```python
from build123d import *

# Parameters (mm, degrees)
AUFSATZ_LINEAR_AUSTRAGEN1_DEPTH      = 3
AUFSATZ_LINEAR_AUSTRAGEN1_DEPTH_BACK = 1
AUFSATZ_LINEAR_AUSTRAGEN3_DEPTH      = 31.65
SCHNITT_LINEAR_AUSTRAGEN1_DEPTH      = 28.65
SKIZZE7_R                            = 2.5
SCHNITT_LINEAR_AUSTRAGEN2_DEPTH      = 110.867294952
SCHNITT_LINEAR_AUSTRAGEN6_DEPTH      = 2
SKIZZE9_R                            = 1
SCHNITT_LINEAR_AUSTRAGEN5_DEPTH      = 13.1
SKIZZE10_R                           = 1.25
SCHNITT_LINEAR_AUSTRAGEN7_DEPTH      = 111.405717696
SKIZZE11_R                           = 2.75
SCHNITT_LINEAR_AUSTRAGEN8_DEPTH      = 1.4


with BuildPart() as part:
    # Skizze2 → Aufsatz-Linear austragen1 (new, two sides: drawn at the far end of the back side and taken through both)
    with BuildSketch(Plane(origin=(0, 0, 0), x_dir=(1, 0, 0), z_dir=(0, 1, 0)).offset(-AUFSATZ_LINEAR_AUSTRAGEN1_DEPTH_BACK)):
        Polygon((-53.033008589, 53.033008589), (0, 0), (53.033008589, 53.033008589), (0, 75), align=None)
        Polygon((53.033008589, 53.033008589), (0, 0), (75, 0), align=None)
        Polygon((75, 0), (0, 0), (53.033008589, -53.033008589), align=None)
        Polygon((53.033008589, -53.033008589), (0, 0), (-53.033008589, -53.033008589), (0, -75), align=None)
        Polygon((-53.033008589, 53.033008589), (-75, 0), (0, 0), align=None)
        Polygon((0, 0), (-75, 0), (-53.033008589, -53.033008589), align=None)
    extrude(amount=AUFSATZ_LINEAR_AUSTRAGEN1_DEPTH + AUFSATZ_LINEAR_AUSTRAGEN1_DEPTH_BACK)

    # Skizze5 → Aufsatz-Linear austragen3 (add)
    with BuildSketch(Plane(origin=(0, 0, 0), x_dir=(1, 0, 0), z_dir=(0, 1, 0))):
        Polygon((20.35, -4), (28.35, -4), (28.35, -11.925), (-28.35, -11.925), (-28.35, 11.925), (28.35, 11.925), (28.35, 4), (20.35, 4), (20.35, 9.925), (-20.35, 9.925), (-20.35, -9.925), (20.35, -9.925), align=None)
    extrude(amount=AUFSATZ_LINEAR_AUSTRAGEN3_DEPTH)

    # Skizze6 → Schnitt-Linear austragen1 (cut)
    with BuildSketch(Plane.XY.offset(11.925)):
        Polygon((-19, 31.65), (19, 31.65), (-2.152730863, 14.994542406), align=None)
    extrude(amount=-SCHNITT_LINEAR_AUSTRAGEN1_DEPTH, mode=Mode.SUBTRACT)

    # Skizze7 → Schnitt-Linear austragen2 (cut, through all)
    with BuildSketch(Plane(origin=(0, 3, 0), x_dir=(1, 0, 0), z_dir=(0, 1, 0))):
        with Locations(Location((35, 40, 0), (0, 0, 270))):
            Circle(SKIZZE7_R)
        with Locations(Location((-35, 40, 0), (0, 0, 270))):
            Circle(SKIZZE7_R)
        with Locations(Location((0, -40, 0), (0, 0, 270))):
            Circle(SKIZZE7_R)
    extrude(amount=-SCHNITT_LINEAR_AUSTRAGEN2_DEPTH, mode=Mode.SUBTRACT)

    # Skizze8 → Schnitt-Linear austragen6 (cut)
    with BuildSketch(Plane(origin=(0, 3, 0), x_dir=(1, 0, 0), z_dir=(0, 1, 0))):
        Polygon((-32.35, 8.05), (-32.35, -8.05), (-49.95, 0), align=None)
        Polygon((32.35, -8.05), (49.95, 0), (32.35, 8.05), align=None)
    extrude(amount=-SCHNITT_LINEAR_AUSTRAGEN6_DEPTH, mode=Mode.SUBTRACT)

    # Skizze9 → Schnitt-Linear austragen5 (cut)
    with BuildSketch(Plane(origin=(0, 31.65, 0), x_dir=(1, 0, 0), z_dir=(0, 1, 0))):
        with Locations(Location((-24.4, -5.375, 0), (0, 0, 270))):
            Circle(SKIZZE9_R)
        with Locations(Location((-24.4, 5.525, 0), (0, 0, 270))):
            Circle(SKIZZE9_R)
        with Locations(Location((24.9, 5.525, 0), (0, 0, 270))):
            Circle(SKIZZE9_R)
        with Locations(Location((24.9, -5.375, 0), (0, 0, 270))):
            Circle(SKIZZE9_R)
    extrude(amount=-SCHNITT_LINEAR_AUSTRAGEN5_DEPTH, mode=Mode.SUBTRACT)

    # Skizze10 → Schnitt-Linear austragen7 (cut, through all)
    with BuildSketch(Plane(origin=(0, 1, 0), x_dir=(1, 0, 0), z_dir=(0, 1, 0))):
        with Locations(Location((-37.437800905, 0, 0), (0, 0, 270))):
            Circle(SKIZZE10_R)
        with Locations(Location((37.44, 0.05, 0), (0, 0, 90))):
            Circle(SKIZZE10_R)
    extrude(amount=-SCHNITT_LINEAR_AUSTRAGEN7_DEPTH, mode=Mode.SUBTRACT)

    # Skizze11 → Schnitt-Linear austragen8 (cut)
    with BuildSketch(Plane.XZ.offset(1)):
        with Locations(Location((-37.437800905, 0, 0), (0, 0, 270))):
            Circle(SKIZZE11_R)
        with Locations(Location((37.44, -0.05, 0), (0, 0, 270))):
            Circle(SKIZZE11_R)
    extrude(amount=-SCHNITT_LINEAR_AUSTRAGEN8_DEPTH, mode=Mode.SUBTRACT)


solid = part.part
```
CAD build for the part. Positions are in the model's coordinates, mm. A direction names the side the tool comes from. Give positions to 0.01 mm unless a question says otherwise; leave off trailing zeros. Order: outer loops, then holes, each group sorted by start corner. A loop starts at its lowest first (then second) coordinate and runs counter-clockwise, first axis right, second up.
(1) Saw through at D-D, the plane z = 40. Give the cut face in (x, y).
(2) Saw through at B-B, the plane z = -40. Give the cut face in (x, y), then the cut area to 3 significant figures.
(3) Flat gauge pins, fed straight in: pin 1 (5 mm diameter, centred on x = 41.5, z = 4, fed in from +Y); pin 2 (1.8 mm diameter, centred on y = 15.5, z = 5.5, fed in from -X); pin 3 (9 mm diameter, centred on x = 25.5, y = 13.5, fed in from +Z) (3 decimals); pin 4 (2 mm diameter, centred on x = -37.44, z = 0, fed in from +Y). Where does each tip first touch, or does it go through?
(4) Mould opens along Z. For faces 5 (the flat face through (20.35, 17, 7)), 6 (the flat face through (-26.15, 0.97, -64.17)), 7 (the flat face through (-10.46, 23.21, 10.94)), 8 (the flat face through (24, 17, -4)) say: released by +Z, released by -Z, zero draft, split by the parting line, or undercut.
(5) Tool access for faces 1 (the flat face through (0, 14, 11.925)), 2 (the flat face through (0, 14, 9.925)), 3 (the flat face through (-10.46, 23.21, -10.91)), 4 (the flat face through (36, 0.4, -1)): list every direction of +Z, -Z, +X, -X, +Y, -Y with a clear straight run to the whole face (end or side of a thin tool).
(6) Saw through at C-C, the plane y = 6. Give the cut face in (x, z) (3 decimals).
(7) Drill centre lines: L1, parallel to X at y = 0, z = 0; L2, parallel to X at y = 20, z = 5.5; L3, parallel to Z at x = 37, y = 0. Where is each one in solid material? Low to high.
(8) Saw through at A-A, the plane y = 26. Give the cut face in (x, z) (3 decimals).
Results found:
1. outline: (-58.43, -1) - (-2.5, -1) - (-2.5, 3) - (-58.43, 3) - close; (2.5, -1) - (58.43, -1) - (58.43, 3) - (2.5, 3) - close
2. outline: (-58.43, -1) - (-37.5, -1) - (-37.5, 3) - (-58.43, 3) - close; (-32.5, -1) - (32.5, -1) - (32.5, 3) - (-32.5, 3) - close; (37.5, -1) - (58.43, -1) - (58.43, 3) - (37.5, 3) - close
2. area: 427 mm2
3. pin 1: stops at y = 3
3. pin 2: stops at x = -28.35
3. pin 3: stops at z = 11.925
3. pin 4: passes through
4. face 5: undercut
4. face 6: released by -Z
4. face 7: zero draft
4. face 8: undercut
5. face 1: +Z, +X, -X, +Y
5. face 2: +Y
5. face 3: +Z, -Z, +Y
5. face 4: -Y
6. outline: (-28.35, -11.925) - (28.35, -11.925) - (28.35, -4) - (20.35, -4) - (20.35, -9.925) - (-20.35, -9.925) - (-20.35, 9.925) - (20.35, 9.925) - (20.35, 4) - (28.35, 4) - (28.35, 11.925) - (-28.35, 11.925) - close
7. L1: x = -75 to -40.19, -34.69 to 34.69, 40.19 to 75
7. L2: x = -28.35 to -25.39, -23.41 to -20.35, 20.35 to 23.91, 25.89 to 28.35
7. L3: z = -59.67 to -41.5, -38.5 to -2.76, 2.66 to 59.67
8. outline: (-28.35, -11.925) - (-13.285, -11.925) - (-13.285, -9.925) - (-20.35, -9.925) - (-20.35, 9.925) - (-13.285, 9.925) - (-13.285, 11.925) - (-28.35, 11.925) - close; (11.824, -11.925) - (28.35, -11.925) - (28.35, -4) - (20.35, -4) - (20.35, -9.925) - (11.824, -9.925) - close; (11.824, 9.925) - (20.35, 9.925) - (20.35, 4) - (28.35, 4) - (28.35, 11.925) - (11.824, 11.925) - close; hole circle Ø2 at (-24.4, -5.525); hole circle Ø2 at (-24.4, 5.375); hole circle Ø2 at (24.9, -5.525); hole circle Ø2 at (24.9, 5.375)
